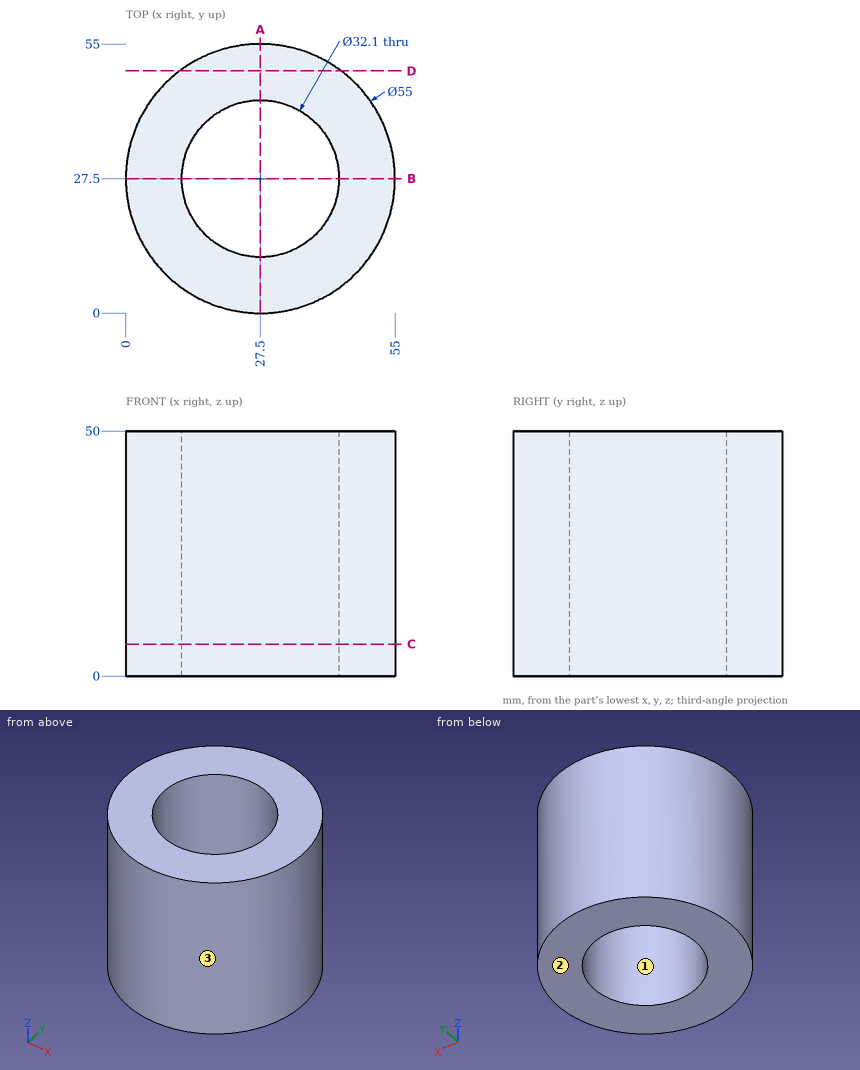
Job drawing, mm, ordinate dimensions from the low corner. One solid piece. Give positions to 0.01 mm unless a question says otherwise; leave off trailing zeros. Write each loop counter-clockwise with the first axis right and the second up, starting at its lowest first coordinate (ties: lowest second). Pieces come first, ordered by that corner, then holes. Notation, with made-up numbers: (1, -21) - (13, -21) arc R20 ccw to (13, 1) - close; hole circle Ø11 at (62.5, -28.75). An arc over 180 degrees is marked (long way). Answer as CSV lines item,"result".
1. Band-saw the part on A-A (x = 27.5). Write the cut outline in (y, z).
Responses:
outline,"(0, 0) - (11.45, 0) - (11.45, 50) - (0, 50) - close; (43.55, 0) - (55, 0) - (55, 50) - (43.55, 50) - close"
2. Drill centre lines: L1, parallel to Y at x = 27.5, z = 31.5; L2, parallel to X at y = 27, z = 39; L3, parallel to X at y = 30, z = 29. Where is each one in solid material? Low to high. Write a range as [from, to].
Responses:
L1,"y = [0, 11.45], [43.55, 55]"
L2,"x = [0, 11.46], [43.54, 55]"
L3,"x = [0.11, 11.65], [43.35, 54.89]"
3. Pin check, flat tips, straight feed: pin 1 (6 mm diameter, centred on x = 37.5, z = 15, fed in from +Y); pin 2 (2 mm diameter, centred on x = 8.5, z = 6, fed in from +Y); pin 3 (10 mm diameter, centred on y = 15.5, z = 17, fed in from +X). Stop position of each tip, or through.
Responses:
pin 1,"stops at y = 54.09"
pin 2,"stops at y = 48.29"
pin 3,"stops at x = 54.09"
4. Band-saw the part on C-C (z = 6.5). Write the cut outline in (x, y).
Responses:
outline,"circle Ø55 at (27.5, 27.5); hole circle Ø32.1 at (27.5, 27.5)"
5. Band-saw the part on D-D (y = 49.5). Write the cut outline in (x, z).
Responses:
outline,"(11, 0) - (44, 0) - (44, 50) - (11, 50) - close"
6. Two-plate mould, pull along Y, no slides. Class the marked faces 1, 2 and 3: +Y half, -Y half, draft (parallel to the pull), parting line (faces both ways), or undercut.
Responses:
face 1,"undercut"
face 2,"draft"
face 3,"parting line"
